Source: three-view drawing plus pictorial views. Frame: mm from the lowest corner of the part. Round coordinates to 2 decimals unless told otherwise and drop trailing zeros. Write each loop counter-clockwise with the first axis right and the second up, starting at its lowest first coordinate (ties: lowest second). Pieces come first, ordered by that corner, then holes. Notation, with made-up numbers: (59, 48) -> (71, 48) arc R17 ccw to (71, 61) -> close; hole circle Ø7 at (15, 86.5). An arc over 180 degrees is marked (long way). Put each result on its own line as item: value.
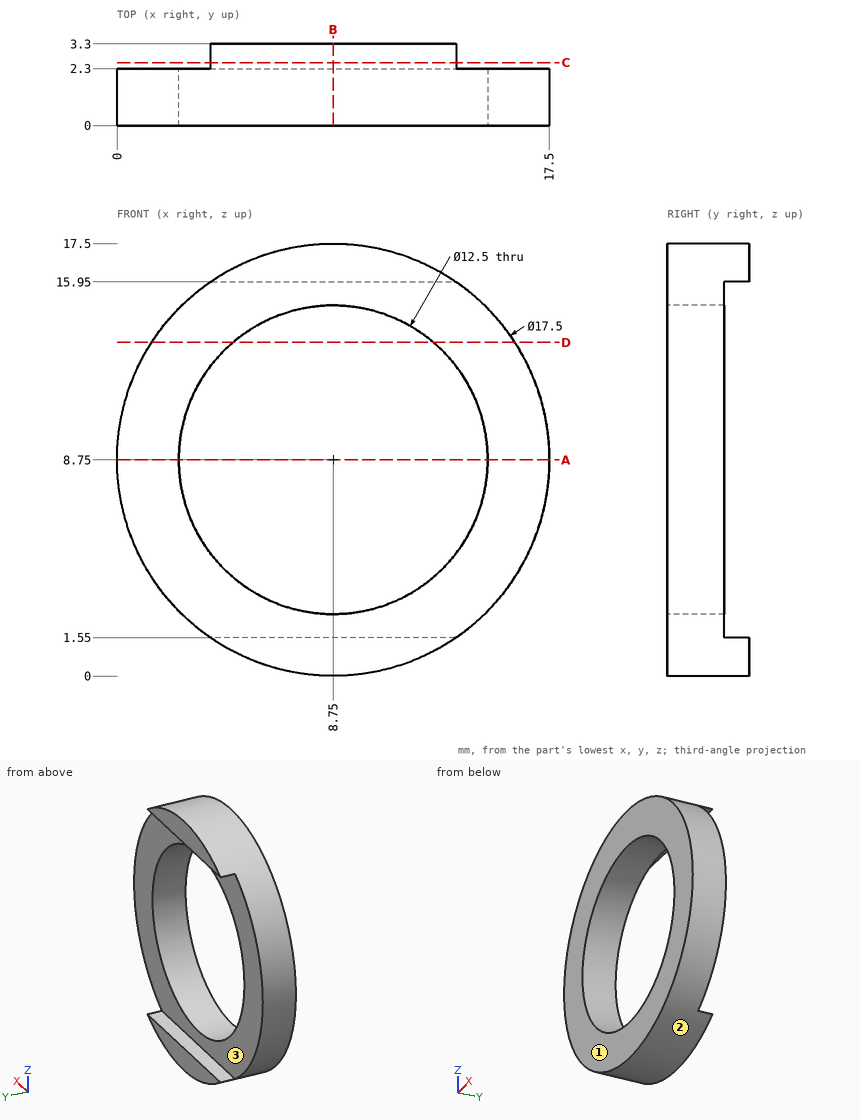
Q1. Pin query (flat end, axial travel): pin 1 (1 mm diameter, centred on x = 2.5, y = 1, fed in from -Z); pin 2 (0.8 mm diameter, centred on x = 7, y = 3, fed in from -Z); pin 3 (1.5 mm diameter, centred on y = 1.5, z = 15, fed in from -X). Return the tip coordinate at first contact, or that it passes through.
Ans:
pin 1: stops at z = 2.15
pin 2: stops at z = 0.1
pin 3: stops at x = 1.94
Q2. Cut plane C-C on y = 2.55. Output: boundary loops of the cut face in (x, z), and give its area (3 significant figures).
Ans:
outline: (3.78, 1.55) arc R8.75 ccw to (13.72, 1.55) -> close; (3.78, 15.95) -> (13.72, 15.95) arc R8.75 ccw to start
area: 20.9 mm^2
Q3. Cut plane A-A on z = 8.75. Output: boundary loops of the cut face in (x, y), and give its area (3 significant figures).
Ans:
outline: (0, 0) -> (2.5, 0) -> (2.5, 2.3) -> (0, 2.3) -> close; (15, 0) -> (17.5, 0) -> (17.5, 2.3) -> (15, 2.3) -> close
area: 11.5 mm^2
Q4. Draft query along Z for the marked faces 1, 2 and 3. Return one class per face: +Z half, -Z half, draft (parallel to the pull), parting line (faces both ways), or undercut.
Ans:
face 1: draft
face 2: parting line
face 3: undercut
Q5. Material intervals for line 1 (X direction, y = 0.8, z = 9) (3 decimals); line 2 (Z direction, x = 8.75, y = 1.5); line 3 (Z direction, x = 7.5, y = 2.15), sorted ascending. Write a range as [from, to].
Ans:
line 1: x = [0.004, 2.505], [14.995, 17.496]
line 2: z = [0, 2.5], [15, 17.5]
line 3: z = [0.09, 2.63], [14.87, 17.41]
Q6. Cut plane D-D on z = 13.5. Output: boundary loops of the cut face in (x, y), and give its area (3 significant figures).
Ans:
outline: (1.4, 0) -> (4.69, 0) -> (4.69, 2.3) -> (1.4, 2.3) -> close; (12.81, 0) -> (16.1, 0) -> (16.1, 2.3) -> (12.81, 2.3) -> close
area: 15.1 mm^2
Q7. Cut plane B-B on x = 8.75. Output: boundary loops of the cut face in (y, z), and give its area (3 significant figures).
Ans:
outline: (0, 0) -> (3.3, 0) -> (3.3, 1.55) -> (2.3, 1.55) -> (2.3, 2.5) -> (0, 2.5) -> close; (0, 15) -> (2.3, 15) -> (2.3, 15.95) -> (3.3, 15.95) -> (3.3, 17.5) -> (0, 17.5) -> close
area: 14.6 mm^2
